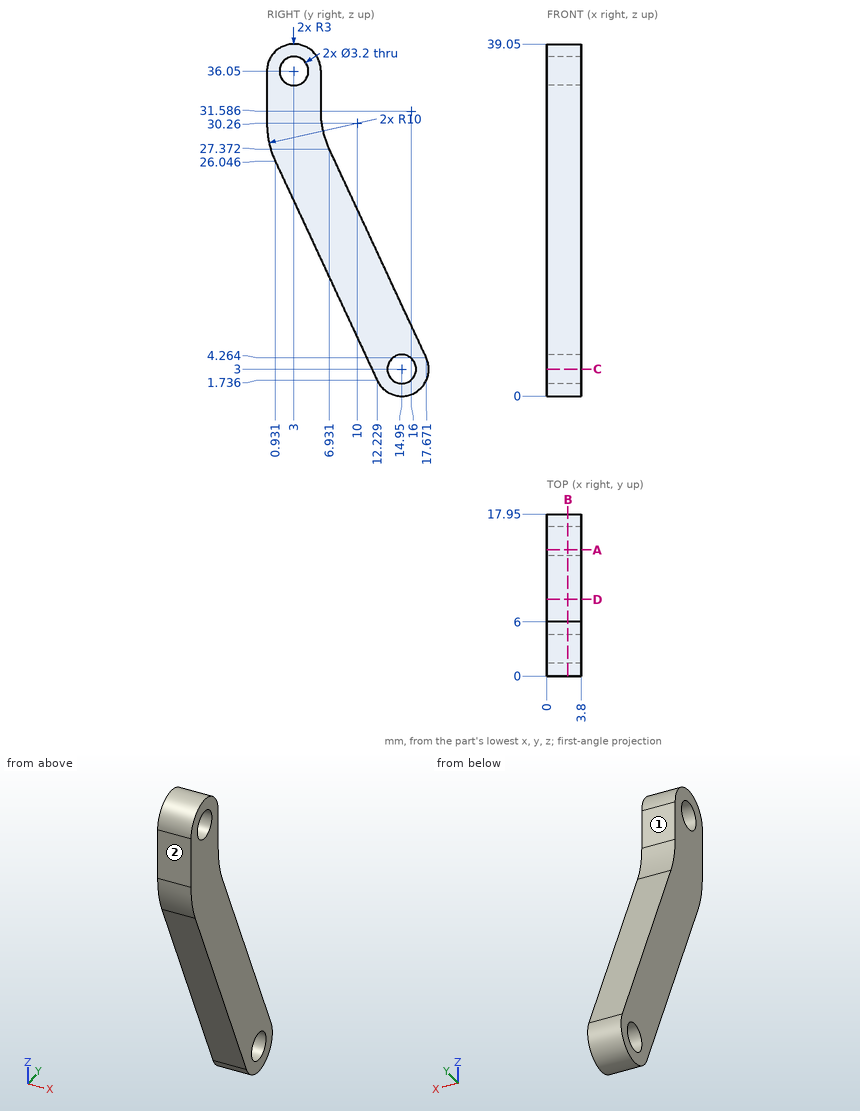
Here's the drawing with two shaded views (mm, measured from the low corner). I have some questions. A direction names the side the tool comes from. Round coordinates to 2 decimals unless told otherwise and drop trailing zeros. Write each loop counter-clockwise with the first axis right and the second up, starting at its lowest first coordinate (ties: lowest second). Pieces come first, ordered by that corner, then holes. Notation, with made-up numbers: M -25,-10.5 L 27,-10.5 A18 ccw 27,0.5 Z; hole C 55.5,-18 d5. An arc over 180 degrees is marked long. Use CSV: the item, a comma, the result in double quotes.
(1) I need wall thicknesses on line 1 along Y through (x, z) = (1.4, 3); line 2 along Z through (x, y) = (2.4, 14.25) (1 decimal); line 3 along Y through (x, z) = (0.3, 10.5) (1 decimal). Which ranges of each line are inside material? Lowest first, please.
Check values:
line 1,"11.64 to 13.35, 16.55 to 17.95"
line 2,"0.1 to 1.6, 4.4 to 11.6"
line 3,"8.2 to 14.8"
(2) On a 3-axis mill with a long thin cutter (end or side, diameter ignored), from which of +Z, -Z, +X, -X, +Y, -Y can I reach the whole of each face in a straight line? I mean the marked faces 1 and 2. Say none if no direction works.
Check values:
face 1,"+Z, +X, -X, +Y"
face 2,"+Z, -Z, +X, -X, -Y"
(3) Imagine slicing it at D-D (y = 8.5). Write out the boundary of the cut face in (x, z), plus the area to 3 significant figures.
Check values:
outline,"M 0,9.76 L 3.8,9.76 L 3.8,24 L 0,24 Z"
area,"54.1 mm^2"
(4) Imagine slicing it at C-C (z = 3). Write out the boundary of the cut face in (x, y), plus the area to 3 significant figures.
Check values:
outline,"M 0,11.64 L 3.8,11.64 L 3.8,13.35 L 0,13.35 Z; M 0,16.55 L 3.8,16.55 L 3.8,17.95 L 0,17.95 Z"
area,"11.8 mm^2"
(5) I'm going to push flat-ended pins straight in: pin 1 (5 mm diameter, centred on y = 6.5, z = 13, fed in from +X); pin 2 (3 mm diameter, centred on y = 3, z = 36.05, fed in from +X); pin 3 (1 mm diameter, centred on x = 1.5, y = 14.5, fed in from +Z) (1 decimal); pin 4 (1.5 mm diameter, centred on x = 3.5, z = 16, fed in from -Y). Where does each tip first touch, or does it pass through?
Check values:
pin 1,"x = 3.8"
pin 2,"through"
pin 3,"z = 12.2"
pin 4,"y = 5.25"
(6) Imagine slicing it at B-B (x = 2.35). Count the separate pieces of the cut face and the enclosed holes in it, plus the area to 3 significant figures.
Check values:
separate pieces,"1"
enclosed holes,"2"
area,"226 mm^2"
(7) Imagine slicing it at A-A (y = 14). Write out the boundary of the cut face in (x, z) (1 decimal).
Check values:
outline,"M 0,0.2 L 3.8,0.2 L 3.8,1.7 L 0,1.7 Z; M 0,4.3 L 3.8,4.3 L 3.8,12.2 L 0,12.2 Z"
